from build123d import *

# Parameters (mm, degrees)
SKETCH2_W           = 22
SKETCH2_H           = 10
SKETCH2_R           = 1.5
BOSS_EXTRUDE1_DEPTH = 2
SKETCH3_W           = 3
SKETCH3_H           = 3
SKETCH3_R           = 1
BOSS_EXTRUDE2_DEPTH = 4
FILLET1_R           = 1.5
FILLET2_R           = 1
FILLET3_R           = 1
FILLET4_R           = 1.5


with BuildPart() as part:
    # Sketch2 → Boss-Extrude1 (new body)
    with BuildSketch(Plane(origin=(0, 0, 0), x_dir=(1, 0, 0), z_dir=(0, 1, 0))):
        Rectangle(SKETCH2_W, SKETCH2_H)
        with Locations(Location((-7.5, 0, 0), (0, 0, 270))):
            Circle(SKETCH2_R, mode=Mode.SUBTRACT)
        with Locations(Location((7.5, 0, 0), (0, 0, 270))):
            Circle(SKETCH2_R, mode=Mode.SUBTRACT)
    extrude(amount=BOSS_EXTRUDE1_DEPTH)

    # Sketch3 → Boss-Extrude2 (add)
    with BuildSketch(Plane(origin=(11, 0, 0), x_dir=(0, 0, -1), z_dir=(1, 0, 0))):
        with Locations((6, 3.5)):
            Rectangle(SKETCH3_W, SKETCH3_H)
        with Locations((6, 3.5)):
            Circle(SKETCH3_R, mode=Mode.SUBTRACT)
    boss_extrude2 = extrude(amount=-BOSS_EXTRUDE2_DEPTH)

    # Mirror1: Boss-Extrude2 across plane
    add(boss_extrude2.mirror(Plane(origin=(0, 0, 0), x_dir=(0, 0, 1), z_dir=(1, 0, 0))))

    # Fillet1
    fillet1_edges = [part.edges().sort_by_distance(p)[0] for p in [
        (9, 5, -7.5),
        (9, 5, -4.5),
        (-9, 5, -7.5),
        (-9, 5, -4.5),
    ]]
    fillet(fillet1_edges, radius=FILLET1_R - 0.0001)  # a hair under: the kernel refuses the full size

    # Fillet2
    fillet2_edges = [part.edges().sort_by_distance(p)[0] for p in [
        (9, 2, -4.5),
        (-9, 2, -4.5),
    ]]
    fillet(fillet2_edges, radius=FILLET2_R)

    # Fillet3
    fillet3_edges = [part.edges().sort_by_distance(p)[0] for p in [
        (-9, 2, -5),
        (9, 2, -5),
    ]]
    fillet(fillet3_edges, radius=FILLET3_R)

    # Fillet4
    fillet4_edges = [part.edges().sort_by_distance(p)[0] for p in [
        (-9, 2, -7.5),
        (9, 2, -7.5),
    ]]
    fillet(fillet4_edges, radius=FILLET4_R - 0.0001)  # a hair under: the kernel refuses the full size


solid = part.part
Check sheet for the modelled part. Datum: model origin and axes. Units: mm. Round coordinates to 2 decimals unless told otherwise and drop trailing zeros. Order: outer loops, then holes, each group sorted by start corner. A loop starts at its lowest first (then second) coordinate and runs counter-clockwise, first axis right, second up. Notation, with made-up numbers: M 16,7 L 25,7 A36 cw 25,43 Z; hole C 87,-27 d11. An arc over 180 degrees is marked long. One line per item, written item: value. Start each with the question number.
1. Section check C-C on y = 2.75. Enter the section's corners in (x, z), and give its area (3 significant figures).
2. Gauge pin test, flat ends, axial feed: P1, Ø5, axis at x = 3, z = 2, coming from the +Y side; P2, Ø3, axis at y = 3, z = -6, coming from the +X side; P3, Ø0.6, axis at x = -5, y = 1, coming from the -Z side. Record the tip position at first contact, or that the pin passes through.
3. Scan lines: line 1 along X through (y, z) = (1.1, 0); line 2 along Y through (x, z) = (-8, -6); line 3 along Y through (x, z) = (5.5, 2.5). Record each from-to range of solid material in increasing order.
4. Release check for a two-part mould opening along Y. For faces 1 (the cylindrical face through (9.028, 1.699, -5.285)), 2 (the flat face through (11, 1, -1)), 3 (the cylindrical face through (9.028, 4.176, -5.263)) record: released by +Y, released by -Y, zero draft, split by the parting line, or undercut.
5. Section check D-D on x = -3.75. Enter the section's corners in (y, z), and give its area (3 significant figures).
6. Section check A-A on x = 7.5. Give the number of separate pieces and of enclosed holes in the cut face, and give its area (3 significant figures).
7. Section check B-B on z = 0. Enter the section's corners in (x, y), and give its area (3 significant figures).
Results found:
1. outline: M -11,-7.3 L -7,-7.3 L -7,-6.66 L -11,-6.66 Z; M -11,-5.34 L -7,-5.34 L -7,-4.47 L -11,-4.47 Z; M 7,-7.3 L 11,-7.3 L 11,-6.66 L 7,-6.66 Z; M 7,-5.34 L 11,-5.34 L 11,-4.47 L 7,-4.47 Z
1. area: 12.1 mm^2
2. P1: y = 2
2. P2: x = 11
2. P3: z = -5
3. line 1: -11 to -9, -6 to 6, 9 to 11
3. line 2: 2 to 2.5, 4.5 to 5
3. line 3: 0 to 2
4. face 1: released by -Y
4. face 2: zero draft
4. face 3: undercut
5. outline: M 0,-5 L 2,-5 L 2,5 L 0,5 Z
5. area: 20.0 mm^2
6. separate pieces: 2
6. enclosed holes: 1
6. area: 18.8 mm^2
7. outline: M -11,0 L -9,0 L -9,2 L -11,2 Z; M -6,0 L 6,0 L 6,2 L -6,2 Z; M 9,0 L 11,0 L 11,2 L 9,2 Z
7. area: 32.0 mm^2
